from build123d import *

# Parameters (mm, degrees)
F0_R     = 1.65
F0_R_2   = 1.6
F1_DEPTH = 3.2


with BuildPart() as f1:
    # F0 (on Top) → F1 (new body)
    with BuildSketch(Plane.XY):
        Polygon((-19.510088, 4.530542), (-50.010088, 4.530542), (-53.210088, 4.530542), (-53.210088, -2.469458), (-50.010088, -2.469458), (-50.010088, -18.335517), (-53.210088, -18.335517), (-53.210088, -25.335517), (-50.010088, -25.469458), (-19.510088, -25.469458), (-16.310088, -25.469458), (-16.310088, -18.469458), (-19.510088, -18.469458), (-19.510088, -2.469458), (-16.310088, -2.469458), (-16.310088, 4.530542), align=None)
        with Locations((-43.710088, -16.469458)):
            Circle(F0_R, mode=Mode.SUBTRACT)
        with Locations((-34.510088, -10.966575)):
            Circle(F0_R, mode=Mode.SUBTRACT)
        with Locations((-34.737864, -1.969458)):
            Circle(F0_R, mode=Mode.SUBTRACT)
        with Locations((-24.019817, -1.966214)):
            Circle(F0_R_2, mode=Mode.SUBTRACT)
    extrude(amount=F1_DEPTH)


solid = f1.part
Here's how the part is built. I have some questions about the finished solid (model axes, mm). A direction names the side the tool comes from. Give positions to 0.01 mm unless a question says otherwise; leave off trailing zeros. Loops run counter-clockwise (first coordinate to the right, second up) from the corner with the lowest first, then second, coordinate; pieces in that order, holes last. Notation, with made-up numbers: (-15.75, 53) -> (19.25, 53) arc R22 cw to (19.25, 67) -> close; hole circle Ø1 at (25, 63). An arc over 180 degrees is marked (long way). Answer as a JSON object with one key per item and string values. Group by question number.
Item 1: Will these pins go through, and if not, where does the flat tip stop? pin 1 (1 mm diameter, centred on x = -51.5, z = 2, fed in from -Y); pin 2 (1 mm diameter, centred on y = -3.5, z = 1, fed in from +X); pin 3 (8 mm diameter, centred on x = -20.5, y = -10.5, fed in from -Z); pin 4 (1.9 mm diameter, centred on x = -24.02, y = -1.97, fed in from -Z).
Item 2: I need wall thicknesses on L1, parallel to X at y = -2.25, z = 3; L2, parallel to Y at x = -18, z = 1.95; L3, parallel to X at y = -13, z = 0.55. Which ranges of each line are inside material? Lowest first, please.
Item 3: On a 3-axis mill with a long thin cutter (end or side, diameter ignored), from which of +Z, -Z, +X, -X, +Y, -Y can I reach the whole of each face in a straight line? I mean faces 5 (the flat face through (-18, -2.469, 2)), 6 (the flat face through (-52, -18.336, 2)), 7 (the flat face through (-35, -7, 0)). Say none if no direction works.
Item 4: Thinking about a two-plate mould opening in X: for faces 1 (the flat face through (-35, -7, 3.2)), 2 (the flat face through (-53.21, -22, 2)), 3 (the cylindrical face through (-36.386, -1.897, 1.578)), 4 (the cylindrical face through (-36.16, -10.89, 1.58)), which applies, pulls with the +X half, pulls with the -X half, needs draft (parallel to the pull), parting line crosses it, or undercut?
Item 5: Imagine slicing it at A-A on x = -19. Write out the boundary of the cut face in (y, z), then the cut area to 3 significant figures.
Item 6: Imagine slicing it at D-D on y = -4.25. Write out the boundary of the cut face in (x, z).
Item 7: Imagine slicing it at C-C on y = -17. Write out the boundary of the cut face in (x, z).
Item 8: Imagine slicing it at B-B on z = 2.25. Write out the boundary of the cut face in (x, y).
Answer list:
{
 "1": {"pin 1": "stops at y = -25.43", "pin 2": "stops at x = -19.51", "pin 3": "stops at z = 0", "pin 4": "passes through"},
 "2": {"L1": "x = -53.21 to -36.36, -33.11 to -25.59, -22.45 to -16.31", "L2": "y = -25.47 to -18.47, -2.47 to 4.53", "L3": "x = -50.01 to -19.51"},
 "3": {"face 5": "+Z, -Z, +X", "face 6": "+Z, -Z, -X", "face 7": "-Z, +X, -X, +Y, -Y"},
 "4": {"face 1": "needs draft", "face 2": "pulls with the -X half", "face 3": "undercut", "face 4": "undercut"},
 "5": {"outline": "(-25.47, 0) -> (-18.47, 0) -> (-18.47, 3.2) -> (-25.47, 3.2) -> close; (-2.47, 0) -> (4.53, 0) -> (4.53, 3.2) -> (-2.47, 3.2) -> close", "area": "44.8 mm2"},
 "6": {"outline": "(-50.01, 0) -> (-19.51, 0) -> (-19.51, 3.2) -> (-50.01, 3.2) -> close"},
 "7": {"outline": "(-50.01, 0) -> (-45.27, 0) -> (-45.27, 3.2) -> (-50.01, 3.2) -> close; (-42.15, 0) -> (-19.51, 0) -> (-19.51, 3.2) -> (-42.15, 3.2) -> close"},
 "8": {"outline": "(-53.21, -25.34) -> (-50.01, -25.47) -> (-16.31, -25.47) -> (-16.31, -18.47) -> (-19.51, -18.47) -> (-19.51, -2.47) -> (-16.31, -2.47) -> (-16.31, 4.53) -> (-53.21, 4.53) -> (-53.21, -2.47) -> (-50.01, -2.47) -> (-50.01, -18.34) -> (-53.21, -18.34) -> close; hole circle Ø3.3 at (-43.71, -16.47); hole circle Ø3.3 at (-34.74, -1.97); hole circle Ø3.3 at (-34.51, -10.97); hole circle Ø3.2 at (-24.02, -1.97)"}
}
